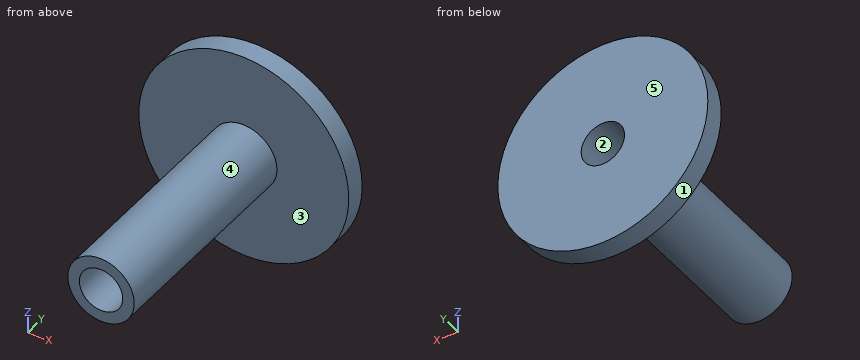
```python
from build123d import *

# Parameters (mm, degrees)
SKETCH1_R           = 7.75
SKETCH1_R_2         = 6.75
BOSS_EXTRUDE1_DEPTH = 1.5
SKETCH2_R           = 1.6
CUT_EXTRUDE3_DEPTH  = 12.062323445
SKETCH5_R           = 2.45
SKETCH5_R_2         = 1.6
BOSS_EXTRUDE3_DEPTH = 16


with BuildPart() as part:
    # Sketch1 → Boss-Extrude1 (new body)
    with BuildSketch(Plane(origin=(0, 0, 0), x_dir=(1, 0, 0), z_dir=(0, 1, 0))):
        with Locations(Location((0, 0, 0), (0, 0, 270))):
            Circle(SKETCH1_R)
        Circle(SKETCH1_R_2, mode=Mode.SUBTRACT)
        Circle(SKETCH1_R_2)
    extrude(amount=BOSS_EXTRUDE1_DEPTH)

    # Sketch2 → Cut-Extrude3 (cut, through all)
    with BuildSketch(Plane(origin=(0, 1.5, 0), x_dir=(1, 0, 0), z_dir=(0, 1, 0))):
        with Locations(Location((0, 0, 0), (0, 0, 270))):
            Circle(SKETCH2_R)
    extrude(amount=-CUT_EXTRUDE3_DEPTH, mode=Mode.SUBTRACT)

    # Sketch5 → Boss-Extrude3 (add)
    with BuildSketch(Plane(origin=(0, 0, 0), x_dir=(-1, 0, 0), z_dir=(0, -1, 0))):
        with Locations(Location((0, 0, 0), (0, 0, 270))):
            Circle(SKETCH5_R)
        with Locations(Location((0, 0, 0), (0, 0, 270))):
            Circle(SKETCH5_R_2, mode=Mode.SUBTRACT)
    extrude(amount=BOSS_EXTRUDE3_DEPTH)


solid = part.part
```
Work out the finished part from the listing and answer in its coordinate system (mm). Face numbers are marked on the shaded views. A direction names the side the tool comes from. Coordinates: 2 decimals unless noted, no trailing zeros. Loops run counter-clockwise (first coordinate to the right, second up) from the corner with the lowest first, then second, coordinate; pieces in that order, holes last.
1) Consider probe 1 along X at (y, z) = (-7.25, 0); probe 2 along Y at (x, z) = (-6, 2.75); probe 3 along Z at (x, y) = (-0.75, -9.75). Determine where each line is inside the solid, lowest interval first.
Results:
probe 1: x = -2.45 to -1.6, 1.6 to 2.45
probe 2: y = 0 to 1.5
probe 3: z = -2.33 to -1.41, 1.41 to 2.33
2) For the marked faces 4 and 5, determine the directions among +Z, -Z, +X, -X, +Y, -Y from which every point of the face is accessible in a straight line to the end or side of a thin tool.
Results:
face 4: -Y
face 5: +Z, -Z, +X, -X, +Y
3) Section D-D (z = -6.25) is taken. Give the vertices of the cut face in (x, y), plus the area to 3 significant figures.
Results:
outline: (-4.58, 0) - (4.58, 0) - (4.58, 1.5) - (-4.58, 1.5) - close
area: 13.7 mm2
4) Section B-B (z = 0) is taken. Give the vertices of the cut face in (x, y).
Results:
outline: (-7.75, 0) - (-2.45, 0) - (-2.45, -16) - (-1.6, -16) - (-1.6, 1.5) - (-7.75, 1.5) - close; (1.6, -16) - (2.45, -16) - (2.45, 0) - (7.75, 0) - (7.75, 1.5) - (1.6, 1.5) - close
5) Flat-ended cylindrical pins translate along their axes: pin 1 (2 mm diameter, centred on y = -4, z = -1, fed in from -X); pin 2 (6 mm diameter, centred on x = 5.5, z = -4, fed in from -Y). Find the tip coordinate at first contact, or state that the pin passes through.
Results:
pin 1: stops at x = -2.45
pin 2: stops at y = 0
6) Section A-A (x = 0) is taken. Give the vertices of the cut face in (y, z), plus the area to 4 significant figures.
Results:
outline: (-16, -2.45) - (0, -2.45) - (0, -7.75) - (1.5, -7.75) - (1.5, -1.6) - (-16, -1.6) - close; (-16, 1.6) - (1.5, 1.6) - (1.5, 7.75) - (0, 7.75) - (0, 2.45) - (-16, 2.45) - close
area: 45.65 mm2
7) For a pull along X with two mould halves and no side action, classify the marked faces 1, 2 and 3 as +X half, -X half, draft (parallel to the pull), parting line (faces both ways), or undercut.
Results:
face 1: parting line
face 2: undercut
face 3: draft
8) Section C-C (y = -10) is taken. Give the vertices of the cut face in (x, z), plus the area to 3 significant figures.
Results:
outline: circle Ø4.9 at (0, 0); hole circle Ø3.2 at (0, 0)
area: 10.8 mm2
